Could you check a few things on this model? Use its own coordinates, in mm. A direction names the side the tool comes from. Coordinates: 2 decimals unless noted, no trailing zeros. Loops run counter-clockwise (first coordinate to the right, second up) from the corner with the lowest first, then second, coordinate; pieces in that order, holes last.
from build123d import *

# Parameters (mm, degrees)
F1_DEPTH = 3.175


with BuildPart() as f1:
    # F0 (on Front) → F1 (new body, symmetric)
    with BuildSketch(Plane.XZ):
        with BuildLine():
            Line((-2.1811367593, -29.9206056496), (0, 0))
            Line((0, 0), (-18.9716252415, -1.0379959996))
            Line((-18.9716252415, -1.0379959996), (-18.560718745, -1.6936484026))
            Line((-18.560718745, -1.6936484026), (-20.6183928033, -29.9206056496))
            ThreePointArc((-20.6183928033, -29.9206056496), (-19.097069056, -35.7098670599), (-14.3476168276, -39.3530356194))
            Line((-14.3476168276, -39.3530356194), (-8.5862497906, -39.3970988002))
            ThreePointArc((-8.5862497906, -39.3970988002), (-6.5372712865, -38.4533368755), (-4.7779318284, -37.0413439039))
            Line((-4.7779318284, -37.0413439039), (23.1049112899, -8.4100140946))
            add(Edge.make_bspline(
                [(23.1049112899, -8.4100140946), (23.9660870284, -7.4624572881), (25.0680023001, -6.8722019142), (25.8537740575, -6.4793160355)],
                knots=[0, 0, 0, 0, 3.3591429725, 3.3591429725, 3.3591429725, 3.3591429725], degree=3))
            Line((25.8537740575, -6.4793160355), (24.10886465, -30.4158005552))
            add(Edge.make_bspline(
                [(24.10886465, -30.4158005552), (23.221265172, -34.8448709212), (26.0528829358, -38.6121878233), (29.4550270257, -39.6880401081)],
                knots=[0, 0, 0, 0, 0.386502628, 0.386502628, 0.386502628, 0.386502628], degree=3))
            Line((29.4550270257, -39.6880401081), (33.3250212912, -39.7176379893))
            add(Edge.make_bspline(
                [(33.3250212912, -39.7176379893), (37.6104290116, -38.509658395), (41.9014469905, -33.599334096), (45.6744432449, -29.5126028359)],
                knots=[0.529238247, 0.529238247, 0.529238247, 0.529238247, 1, 1, 1, 1], degree=3))
            Line((45.6744432449, -29.5126028359), (43.2580737253, -29.0605745563))
            Line((43.2580737253, -29.0605745563), (44.8575740155, -7.1187970799))
            ThreePointArc((44.8575740155, -7.1187970799), (40.634142354, 1.3214875027), (31.2014035881, 1.6364767216))
            add(Edge.make_bspline(
                [(23.4220137692, -5.7100140946), (25.4793688655, -2.7494623791), (28.2295402139, 0), (31.2014035881, 1.6364767216)],
                knots=[0, 0, 0, 0, 10.6999922087, 10.6999922087, 10.6999922087, 10.6999922087], degree=3))
            Line((23.4220137692, -5.7100140946), (23.8800524886, 0.5733130918))
            Line((23.8800524886, 0.5733130918), (4.9084272471, -0.4646829078))
            Line((4.9084272471, -0.4646829078), (5.3193337437, -1.1203353108))
            Line((5.3193337437, -1.1203353108), (3.7198334535, -23.0621127871))
            add(Edge.make_bspline(
                [(3.7198334535, -23.0621127871), (2.6201102883, -25.5734715611), (1.7430323642, -27.2203981876), (-2.1811367593, -29.9206056496)],
                knots=[0, 0, 0, 0, 9.0476722861, 9.0476722861, 9.0476722861, 9.0476722861], degree=3))
        make_face()
        with BuildLine():
            Line((-8.5862497906, -39.3970988002), (-14.3476168276, -39.3530356194))
            ThreePointArc((-14.3476168276, -39.3530356194), (-11.4704542579, -39.8354397482), (-8.5862497906, -39.3970988002))
        make_face()
        with BuildLine():
            Line((33.3250212912, -39.7176379893), (29.4550270257, -39.6880401081))
            add(Edge.make_bspline(
                [(29.4550270257, -39.6880401081), (30.0021087518, -39.8610425176), (31.2924032253, -40.0985217153), (32.5914536336, -39.9244175584), (33.3250212912, -39.7176379893)],
                knots=[0.386502628, 0.386502628, 0.386502628, 0.386502628, 0.4486541769, 0.529238247, 0.529238247, 0.529238247, 0.529238247], degree=3))
        make_face()
        with BuildLine():
            ThreePointArc((-8.5862497906, -39.3970988002), (-11.4704542579, -39.8354397482), (-14.3476168276, -39.3530356194))
            Line((-14.3476168276, -39.3530356194), (-57.49016349, -39.0230795821))
            Line((-57.49016349, -39.0230795821), (-57.747233247, -72.6355695398))
            Line((-57.747233247, -72.6355695398), (80.3876109421, -73.6920307208))
            Line((80.3876109421, -73.6920307208), (80.3876109421, -40.0775746826))
            Line((80.3876109421, -40.0775746826), (33.3250212912, -39.7176379893))
            add(Edge.make_bspline(
                [(29.4550270257, -39.6880401081), (30.0021087518, -39.8610425176), (31.2924032253, -40.0985217153), (32.5914536336, -39.9244175584), (33.3250212912, -39.7176379893)],
                knots=[0.386502628, 0.386502628, 0.386502628, 0.386502628, 0.4486541769, 0.529238247, 0.529238247, 0.529238247, 0.529238247], degree=3))
            Line((29.4550270257, -39.6880401081), (-8.5862497906, -39.3970988002))
        make_face()
    extrude(amount=F1_DEPTH, both=True)


solid = f1.part
(1) Imagine slicing it at A-A, the plane x = 9. Write out the boundary of the cut face in (y, z) (3 decimals).
Answers:
outline: (-3.175, -73.146) - (3.175, -73.146) - (3.175, -39.532) - (-3.175, -39.532) - close; (-3.175, -22.894) - (3.175, -22.894) - (3.175, -0.241) - (-3.175, -0.241) - close
(2) For pin 1 (2 mm diameter, centred on x = -12, y = 2, fed in from -Z); pin 2 (1.5 mm diameter, centred on y = -1, z = -6, fed in from +X); pin 3 (1 mm diameter, centred on y = -2.5, z = -56, fed in from -X), each with a flat end and sliding along its axis, tell me the tip position at first contact or that it passes through.
Answers:
pin 1: stops at z = -72.99
pin 2: stops at x = 44.88
pin 3: stops at x = -57.62
(3) We'd pull the mould along Z, two halves only. Please class faces 6 (the face through (14.53, -0.04, 0.06)), 7 (the face through (-19.144, -0.044, -35.639)), 8 (the face through (10, -3.175, -43)): +Z half, -Z half, draft (parallel to the pull), parting line (faces both ways), or undercut.
Answers:
face 6: +Z half
face 7: undercut
face 8: draft
(4) Which directions (+Z, -Z, +X, -X, +Y, -Y) give clear straight access to the entire face, cutting with the end or side of a thin tool? Please do faces 1 (the face through (-19.575, -0.044, -15.61)), 2 (the face through (-9.35, -0.04, -0.51)), 3 (the face through (44.48, -0.04, -29.29)), 4 (the face through (80.388, 0, -57)), 5 (the face through (-1.106, -0.044, -15.17)).
Answers:
face 1: -X, +Y, -Y
face 2: +Z, -X, +Y, -Y
face 3: +X, +Y, -Y
face 4: +Z, -Z, +X, +Y, -Y
face 5: +Y, -Y
(5) I need wall thicknesses on probe 1 along X at (y, z) = (1.25, -27); probe 2 along X at (y, z) = (-1, -18); probe 3 along X at (y, z) = (0.5, -43). Which ranges of each line are inside material? Lowest first, please.
Answers:
probe 1: x = -20.41 to -1.97, 1.33 to 5, 24.36 to 43.41
probe 2: x = -19.75 to -1.31, 4.09 to 13.77, 25.01 to 44.06
probe 3: x = -57.52 to 80.39
(6) Imagine slicing it at B-B, the plane z = -24.5. State how many separate pieces and enclosed holes the cut face has, and give its area (3 significant figures).
Answers:
separate pieces: 3
enclosed holes: 0
area: 266 mm2
(7) Imagine slicing it at C-C, the plane x = 50.5. Write out the boundary of the cut face in (y, z) (3 decimals), and give its area (3 significant figures).
Answers:
outline: (-3.175, -73.463) - (3.175, -73.463) - (3.175, -39.849) - (-3.175, -39.849) - close
area: 213 mm2
